```python
from build123d import *

# Parameters (mm, degrees)
SKETCH3_W             = 2.5
SKETCH3_H             = 66.4
CORTE_EXTRUS_O1_DEPTH = 22
CHANFRO1_SIZE         = 0.5


with BuildPart() as part:
    # Sketch3 → Revolve2 (revolve)
    with BuildSketch(Plane(origin=(0, 0, 0), x_dir=(0, 0, -1), z_dir=(1, 0, 0)), mode=Mode.PRIVATE) as revolve2_sk:
        with Locations((1.25, 0)):
            Rectangle(SKETCH3_W, SKETCH3_H)
    revolve(revolve2_sk.sketch.rotate(Axis((0, 33.2, 0), (0, -1, 0)), 180), axis=Axis((0, 33.2, 0), (0, -1, 0)))

    # Esboço1 → Corte-extrusão1 (cut)
    with BuildSketch(Plane(origin=(0, 33.2, 0), x_dir=(1, 0, 0), z_dir=(0, 1, 0))):
        with BuildLine():
            Line((-1.5, 2), (1.5, 2))
            ThreePointArc((1.5, 2), (0, 2.5), (-1.5, 2))
        make_face()
    extrude(amount=-CORTE_EXTRUS_O1_DEPTH, mode=Mode.SUBTRACT)

    # Chanfro1
    chanfro1_edges = [part.edges().sort_by_distance(p)[0] for p in [
        (0, -33.2, -2.5),
        (2.371708245, 33.2, 0.790569415),
    ]]
    chamfer(chanfro1_edges, length=CHANFRO1_SIZE - 0.0001)  # a hair under: the kernel refuses the full size


solid = part.part
```
Can you work these out from the model? Positions are in its coordinate system, mm. A direction names the side the tool comes from. Coordinates: 2 decimals unless noted, no trailing zeros. Write each loop counter-clockwise with the first axis right and the second up, starting at its lowest first coordinate (ties: lowest second). Pieces come first, ordered by that corner, then holes. Notation, with made-up numbers: M 73.25,43 L 90.25,43 A30 cw 90.25,72 Z; hole C 81,39.25 d11. An arc over 180 degrees is marked long. Answer as CSV lines item,"result".
Item 1: On a 3-axis mill with a long thin cutter (end or side, diameter ignored), from which of +Z, -Z, +X, -X, +Y, -Y can I reach the whole of each face in a straight line? I mean faces 1 (the flat face through (0, 22, -2)), 2 (the flat face through (0, -33.2, 0)). Say none if no direction works.
Geometry results:
face 1,"-Z, +X, -X, +Y"
face 2,"+Z, -Z, +X, -X, -Y"
Item 2: Imagine slicing it at A-A on y = 20.5. List the corners of the cut face in (x, z) for me.
Geometry results:
outline,"M -1.5,-2 L 1.5,-2 A2.5 ccw long Z"
Item 3: I'm going to push flat-ended pins straight in: P1, Ø1, axis at x = 1.5, y = -16, coming from the +Z side; P2, Ø1.5, axis at x = 0, y = 22, coming from the -Z side. Where does each tip first touch, or does it pass through?
Geometry results:
P1,"stops at z = 2.29"
P2,"stops at z = -2"
Item 4: Please list where these lines run through material, in increasing order: line 1 along Z through (x, y) = (0.2, -6.5); line 2 along X through (y, z) = (30, -1.95).
Geometry results:
line 1,"z = -2.49 to 2.49"
line 2,"x = -1.56 to 1.56"
Item 5: Imagine slicing it at B-B on y = -9.5. List the corners of the cut face in (x, z) for me, plus the area to 3 significant figures.
Geometry results:
outline,"C 0,0 d5"
area,"19.6 mm2"
